For this review, use the dimensioned drawing (mm, ordinates from the lowest corner) and the shaded views. A direction names the side the tool comes from. Coordinates: 2 decimals unless noted, no trailing zeros. Loops run counter-clockwise (first coordinate to the right, second up) from the corner with the lowest first, then second, coordinate; pieces in that order, holes last. Notation, with made-up numbers: M -5.75,73 L 17.25,73 A18 cw 17.25,98 Z; hole C -19.5,57.5 d7. An arc over 180 degrees is marked long. Write item = value, one per line.
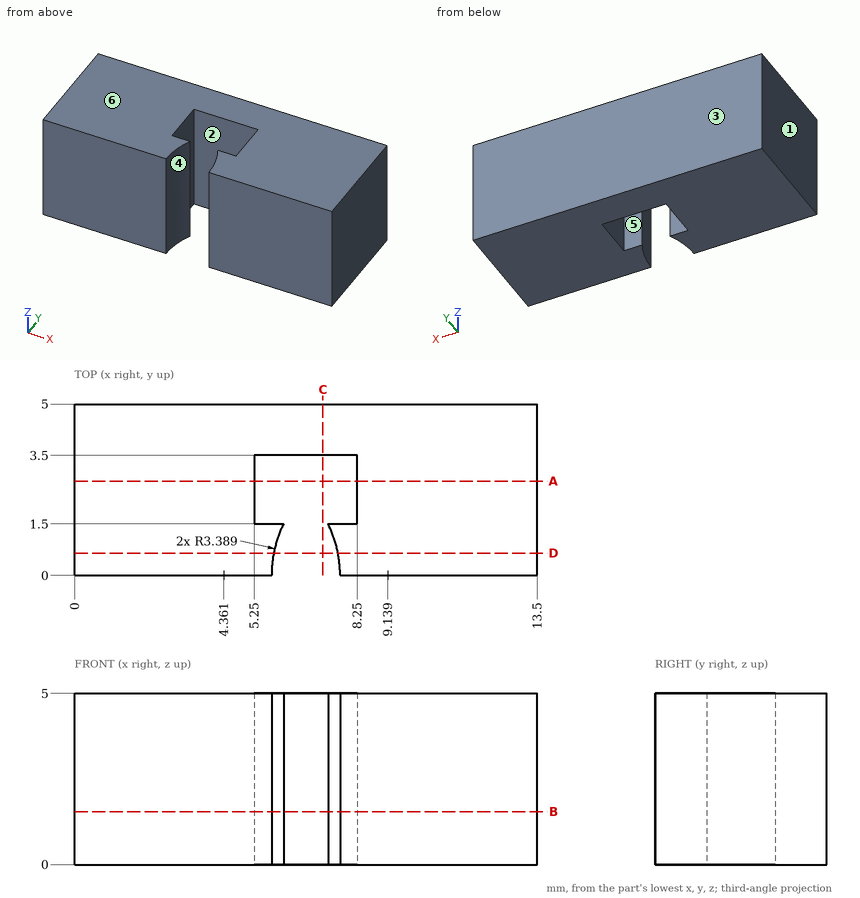
Q1. Add section D-D (y = 0.65). Write out the cut boundary in (x, z).
Solved:
outline = M 0,0 L 5.81,0 L 5.81,5 L 0,5 Z; M 7.69,0 L 13.5,0 L 13.5,5 L 7.69,5 Z
Q2. Machinability: for the marked faces 1 and 2, which of the approach directions +Z, -Z, +X, -X, +Y, -Y give a long, thin tool a straight path to every point of the face, cutting with its end or side? Answer none if there is none.
Solved:
face_1 = +Z, -Z, -X, +Y, -Y
face_2 = +Z, -Z
Q3. For pin 1 Ø1.5 at (y, z) = (2.5, 1.5) entering from -X, flat-tipped, find the tip position at first contact; note if it passes through.
Solved:
pin_1 = 0
Q4. Add section C-C (x = 7.25). Write out the cut boundary in (y, z).
Solved:
outline = M 3.5,0 L 5,0 L 5,5 L 3.5,5 Z
Q5. For line 1 along Y through (x, z) = (5.5, 3); line 2 along X through (y, z) = (2.85, 0.2); line 3 along X through (y, z) = (0.9, 4.3), list the stretches that pass through material, from the lowest coordinate up.
Solved:
line_1 = 0 to 1.5, 3.5 to 5
line_2 = 0 to 5.25, 8.25 to 13.5
line_3 = 0 to 5.87, 7.63 to 13.5
Q6. Add section B-B (z = 1.55). Write out the cut boundary in (x, y).
Solved:
outline = M 0,0 L 5.75,0 A3.39 cw 6.1,1.5 L 5.25,1.5 L 5.25,3.5 L 8.25,3.5 L 8.25,1.5 L 7.4,1.5 A3.39 cw 7.75,0 L 13.5,0 L 13.5,5 L 0,5 Z
Q7. Draft analysis for pull direction Y (two halves, no side actions). For the marked faces 3, 4, 5 and 6, state which applies: +Y half, -Y half, draft (parallel to the pull), parting line (faces both ways), or undercut.
Solved:
face_3 = +Y half
face_4 = -Y half
face_5 = undercut
face_6 = draft
Q8. Add section A-A (y = 2.75). Write out the cut boundary in (x, z).
Solved:
outline = M 0,0 L 5.25,0 L 5.25,5 L 0,5 Z; M 8.25,0 L 13.5,0 L 13.5,5 L 8.25,5 Z
